Build history of the part. All positions in model axes, mm. Face numbers are marked on the shaded views. A direction names the side the tool comes from. Give positions to 0.01 mm unless a question says otherwise; leave off trailing zeros. Loops run counter-clockwise (first coordinate to the right, second up) from the corner with the lowest first, then second, coordinate; pieces in that order, holes last. Notation, with made-up numbers: (16, -9) -> (50, -9) arc R29 cw to (50, 22) -> close; hole circle Ø9 at (50.5, -40). An arc over 180 degrees is marked (long way). One line per question, with ' | ' between items. Start each with the question number.
(1) Flat gauge pins, fed straight in: pin 1 Ø6 at (x, y) = (32, -26.5) entering from +Z; pin 2 Ø17 at (x, y) = (43.5, 2) entering from -Z; pin 3 Ø1.5 at (x, z) = (38, 65) entering from -Y. Where does each tip first touch, or does it go through?
(2) Slice it at D-D, the plane x = 0.5. Write the cut outline in (y, z), then the cut area to 3 significant figures.
(3) Drill centre lines: L1, parallel to X at y = -31, z = 35; L2, parallel to Z at x = -38, y = 62; L3, parallel to Z at x = 35, y = 8. Where is each one in solid material? Low to high. Write a range as from..to.
(4) Slice it at A-A, the plane z = 22.5. Write the cut outline in (x, y), then the cut area to 3 significant figures.
(5) Mould opens along Y. For the marked faces 1, 2 and 3 say: pulls with the +Y half, pulls with the -Y half, needs draft (parallel to the pull), parting line crosses it, or undercut.
(6) Slice it at C-C, the plane y = -7. Write the cut outline in (x, z), then the cut area to 3 significant figures.
(7) 3-axis set-ups, long thin cutter, end or side, ignore diameter. For the marked faces 4, 5 and 6: which of +Z, -Z, +X, -X, +Y, -Y reach the whole face in a straight line?
(8) Slice it at B-B, the plane z = 38.5. Write the cut outline in (x, y), then the cut area to 3 significant figures.
```python
from build123d import *

# Parameters (mm, degrees)
F0_W     = 112.6851290464
F0_H     = 118.5585707426
F1_DEPTH = 101.6
F2_W     = 112.6851290464
F2_H     = 89.7236950696
F3_DEPTH = 50.8
F4_W     = 85.5996385217
F4_H     = 40.2484461665
F5_DEPTH = 127
F6_W     = 72.8077031672
F6_H     = 35.5043448508
F7_DEPTH = 127


with BuildPart() as f1:
    # F0 (on Top) → F1 (new body)
    with BuildSketch(Plane.XY):
        with Locations((-3.3229105175, 13.3671686053)):
            Rectangle(F0_W, F0_H)
    extrude(amount=F1_DEPTH)

    # F2 (on face) → F3 (cut)
    with BuildSketch(Plane.XY.offset(101.6)):
        with Locations((-3.3229105175, -1.0502692312)):
            Rectangle(F2_W, F2_H)
    extrude(amount=-F3_DEPTH, mode=Mode.SUBTRACT)

    # F4 (on face) → F5 (cut)
    with BuildSketch(Plane.XZ.offset(45.912116766)):
        with Locations((-5.4014250636, 20.1242230833)):
            Rectangle(F4_W, F4_H)
    extrude(amount=-F5_DEPTH, mode=Mode.SUBTRACT)

    # F6 (on face) → F7 (cut)
    with BuildSketch(Plane.YZ.offset(53.0196540058)):
        with Locations((11.0908616334, 17.7521724254)):
            Rectangle(F6_W, F6_H)
    extrude(amount=-F7_DEPTH, mode=Mode.SUBTRACT)


solid = f1.part
```
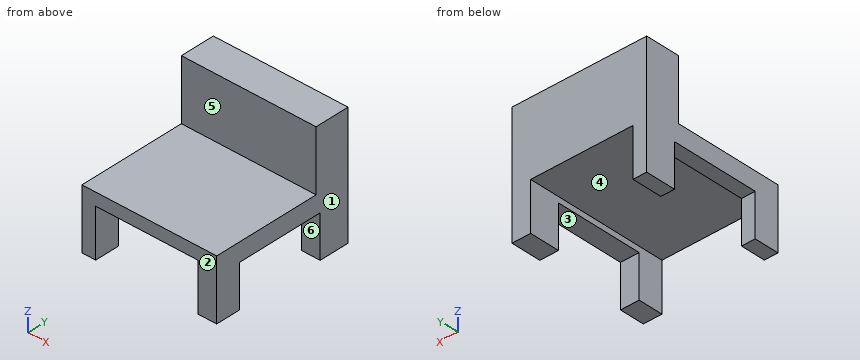
Final values:
1) pin 1: z = 50.8 | pin 2: z = 35.5 | pin 3: y = 43.81
2) outline: (-45.91, 40.25) -> (72.65, 40.25) -> (72.65, 101.6) -> (43.81, 101.6) -> (43.81, 50.8) -> (-45.91, 50.8) -> close | area: 2,720 mm2
3) L1: -59.67..-48.2, 37.4..53.02 | L2: 40.25..101.6 | L3: 40.25..50.8
4) outline: (-59.67, -45.91) -> (-48.2, -45.91) -> (-48.2, -25.31) -> (-59.67, -25.31) -> close; (-59.67, 47.49) -> (-48.2, 47.49) -> (-48.2, 72.65) -> (-59.67, 72.65) -> close; (37.4, -45.91) -> (53.02, -45.91) -> (53.02, -25.31) -> (37.4, -25.31) -> close; (37.4, 47.49) -> (53.02, 47.49) -> (53.02, 72.65) -> (37.4, 72.65) -> close | area: 1,240 mm2
5) face 1: needs draft | face 2: pulls with the -Y half | face 3: undercut
6) outline: (-59.67, 35.5) -> (-48.2, 35.5) -> (-48.2, 40.25) -> (37.4, 40.25) -> (37.4, 35.5) -> (53.02, 35.5) -> (53.02, 50.8) -> (-59.67, 50.8) -> close | area: 1,320 mm2
7) face 4: -Z, +Y, -Y | face 5: +Z, +X, -X, -Y | face 6: -Z, +X, -X
8) outline: (-59.67, -45.91) -> (-48.2, -45.91) -> (-48.2, 72.65) -> (-59.67, 72.65) -> close; (37.4, -45.91) -> (53.02, -45.91) -> (53.02, 72.65) -> (37.4, 72.65) -> close | area: 3,210 mm2
